```python
from build123d import *

# Parameters (mm, degrees)
SKETCH_1_R      = 1.65
EXTRUDE_1_DEPTH = 1.2
SKETCH_2_W      = 17.6
SKETCH_2_H      = 16
SKETCH_2_W_2    = 26.5
SKETCH_2_H_2    = 19.9
EXTRUDE_2_DEPTH = 2.3
SKETCH_3_W      = 17.6
SKETCH_3_H      = 16
EXTRUDE_3_DEPTH = 0.75
SKETCH_5_W      = 37.9
SKETCH_5_H      = 2.5
EXTRUDE_4_DEPTH = 2.45
SKETCH_6_W      = 36.7
SKETCH_6_H      = 0.6
EXTRUDE_5_DEPTH = 5.5


with BuildPart() as part:
    # 草图1 → 凸台-拉伸1 (new body)
    with BuildSketch(Plane.XY):
        with BuildLine():
            Line((0, -2.9), (57.7, -2.9))
            ThreePointArc((57.7, -2.9), (59.750609665, -2.050609665), (60.6, 0))
            Line((60.6, 0), (60.6, 24.1))
            ThreePointArc((60.6, 24.1), (59.750609665, 26.150609665), (57.7, 27))
            Line((57.7, 27), (0, 27))
            ThreePointArc((0, 27), (-2.050609665, 26.150609665), (-2.9, 24.1))
            Line((-2.9, 24.1), (-2.9, 0))
            ThreePointArc((-2.9, 0), (-2.050609665, -2.050609665), (0, -2.9))
        make_face()
        Circle(SKETCH_1_R, mode=Mode.SUBTRACT)
        with Locations((57.7, 0)):
            Circle(SKETCH_1_R, mode=Mode.SUBTRACT)
        with Locations((57.7, 24.1)):
            Circle(SKETCH_1_R, mode=Mode.SUBTRACT)
        with Locations((0, 24.1)):
            Circle(SKETCH_1_R, mode=Mode.SUBTRACT)
    extrude(amount=EXTRUDE_1_DEPTH)

    # 草图2 → 凸台-拉伸2 (add)
    with BuildSketch(Plane(origin=(0, 0, 0), x_dir=(-1, 0, 0), z_dir=(0, 0, -1))):
        with Locations((-45.55, 12.05)):
            Rectangle(SKETCH_2_W, SKETCH_2_H)
        with Locations((-19.85, 14.05)):
            Rectangle(SKETCH_2_W_2, SKETCH_2_H_2)
    extrude(amount=EXTRUDE_2_DEPTH)

    # 草图3 → 凸台-拉伸3 (add)
    with BuildSketch(Plane(origin=(0, 0, -2.3), x_dir=(-1, 0, 0), z_dir=(0, 0, -1))):
        with Locations((-45.55, 12.05)):
            Rectangle(SKETCH_3_W, SKETCH_3_H)
    extrude(amount=EXTRUDE_3_DEPTH)

    # 草图5 → 凸台-拉伸4 (add)
    with BuildSketch(Plane.XY.offset(1.2)):
        with Locations((31.75, 25.75)):
            Rectangle(SKETCH_5_W, SKETCH_5_H)
        with Locations((31.75, -1.65)):
            Rectangle(SKETCH_5_W, SKETCH_5_H)
    extrude(amount=EXTRUDE_4_DEPTH)

    # 草图6 → 凸台-拉伸5 (add)
    with BuildSketch(Plane.XY.offset(3.65)):
        with Locations((31.75, -1.65)):
            Rectangle(SKETCH_6_W, SKETCH_6_H)
        with Locations((31.75, 25.75)):
            Rectangle(SKETCH_6_W, SKETCH_6_H)
    extrude(amount=EXTRUDE_5_DEPTH)


solid = part.part
```
Geometry: final body of the model. Coordinates: model frame, mm. A direction names the side the tool comes from. Round coordinates to 2 decimals unless told otherwise and drop trailing zeros. Order: outer loops, then holes, each group sorted by start corner. A loop starts at its lowest first (then second) coordinate and runs counter-clockwise, first axis right, second up. Notation, with made-up numbers: (-37, -26.5) -> (20, -26.5) arc R25 ccw to (20, -9.5) -> close; hole circle Ø11 at (74, -27.5). An arc over 180 degrees is marked (long way). Use one line per item in the form item = value.
(1) Section A-A on z = 7. Return loops of the section in (x, y), and give its area (3 significant figures).
Results list:
outline = (13.4, -1.95) -> (50.1, -1.95) -> (50.1, -1.35) -> (13.4, -1.35) -> close; (13.4, 25.45) -> (50.1, 25.45) -> (50.1, 26.05) -> (13.4, 26.05) -> close
area = 44.0 mm^2
(2) Section D-D on y = 1. Return loops of the section in (x, z), and give its area (3 significant figures).
Results list:
outline = (-2.9, 0) -> (-1.31, 0) -> (-1.31, 1.2) -> (-2.9, 1.2) -> close; (1.31, 0) -> (56.39, 0) -> (56.39, 1.2) -> (1.31, 1.2) -> close; (59.01, 0) -> (60.6, 0) -> (60.6, 1.2) -> (59.01, 1.2) -> close
area = 69.9 mm^2
(3) Ray query, probe 1 along Y at (x, z) = (57.7, 0.5); probe 2 along Y at (x, z) = (38, 3); probe 3 along Y at (x, z) = (22, 6.5). Return the intervals inside material, ascending. Write a range as [from, to].
Results list:
probe_1 = [-2.9, -1.65], [1.65, 22.45], [25.75, 27]
probe_2 = [-2.9, -0.4], [24.5, 27]
probe_3 = [-1.95, -1.35], [25.45, 26.05]
(4) First-contact query: pin 1 Ø1.5 at (x, z) = (48.5, -1.5) entering from +Y; pin 2 Ø3 at (x, z) = (27.5, 5.5) entering from +Y; pin 3 Ø10 at (x, y) = (30, 12.5) entering from -Z; pin 4 Ø2 at (x, y) = (57.7, 0) entering from -Z. Flat tips, straight axial feed; report the tip coordinate or a pass-through.
Results list:
pin_1 = 20.05
pin_2 = 26.05
pin_3 = -2.3
pin_4 = through
(5) Section C-C on y = 17.25. Return loops of the section in (x, z), and give its area (3 significant figures).
Results list:
outline = (-2.9, 0) -> (6.6, 0) -> (6.6, -2.3) -> (33.1, -2.3) -> (33.1, 0) -> (36.75, 0) -> (36.75, -3.05) -> (54.35, -3.05) -> (54.35, 0) -> (60.6, 0) -> (60.6, 1.2) -> (-2.9, 1.2) -> close
area = 191 mm^2
(6) Access query for faces 4 (the face through (31, 24.5, 2)), 5 (the face through (46, 20.05, -2)), 6 (the face through (54.35, 12, -2)), 7 (the face through (50.7, 26, 2)). Directions: +Z, -Z, +X, -X, +Y, -Y. A direction counts if a zero-diameter tool reaches every point of the face in a straight line with its end or side. Return the directions, or none.
Results list:
face_4 = +Z, +X, -X
face_5 = -Z, +X, +Y
face_6 = -Z, +X, +Y, -Y
face_7 = +Z, +X, +Y, -Y
(7) Draft query along X for faces 1 (the face through (28, -2.9, 2)), 2 (the face through (-2, 26.2, 0.6)), 3 (the face through (56.05, 0.07, 0.59)). Return one class per face: pulls with the +X half, pulls with the -X half, needs draft (parallel to the pull), parting line crosses it, or undercut.
Results list:
face_1 = needs draft
face_2 = pulls with the -X half
face_3 = undercut
(8) Section B-B on x = 43. Return loops of the section in (y, z), and give its area (3 significant figures).
Results list:
outline = (-2.9, 0) -> (4.05, 0) -> (4.05, -3.05) -> (20.05, -3.05) -> (20.05, 0) -> (27, 0) -> (27, 3.65) -> (26.05, 3.65) -> (26.05, 9.15) -> (25.45, 9.15) -> (25.45, 3.65) -> (24.5, 3.65) -> (24.5, 1.2) -> (-0.4, 1.2) -> (-0.4, 3.65) -> (-1.35, 3.65) -> (-1.35, 9.15) -> (-1.95, 9.15) -> (-1.95, 3.65) -> (-2.9, 3.65) -> close
area = 104 mm^2
